from build123d import *

# Parameters (mm, degrees)
F0_R     = 15.6845
F0_R_2   = 11.499076
F1_DEPTH = 12.7
F2_R     = 17.145
F3_DEPTH = 5.08
F5_D     = 0.254


with BuildPart() as f1:
    # F0 (on Top) → F1 (new body)
    with BuildSketch(Plane.XY):
        Circle(F0_R)
        Circle(F0_R_2, mode=Mode.SUBTRACT)
    extrude(amount=F1_DEPTH)

    # F2 (on Top) → F3 (join)
    with BuildSketch(Plane.XY):
        Circle(F2_R)
    extrude(amount=F3_DEPTH)

    # F5 (through all)
    with Locations(Plane.XY.offset(5.08)):
        with Locations((0, 0)):
            Hole(F5_D / 2)


solid = f1.part
Build history of the part. All positions in model axes, mm. A direction names the side the tool comes from. Coordinates: 2 decimals unless noted, no trailing zeros. Order: outer loops, then holes, each group sorted by start corner. A loop starts at its lowest first (then second) coordinate and runs counter-clockwise, first axis right, second up. Notation, with made-up numbers: (60.5, -31.75) - (99.5, -31.75) arc R17 cw to (99.5, -25.75) - close; hole circle Ø1 at (-7, 3). An arc over 180 degrees is marked (long way). Put each result on its own line as item: value.
1. Saw through at A-A (z = 3.5). Write the cut outline in (x, y) (3 decimals).
Answer sheet:
outline: circle Ø34.29 at (0, 0); hole circle Ø0.254 at (0, 0)
2. Drop flat-ended pins along their axis: P1, Ø5, axis at x = -10, z = 6.5, coming from the -Y side; P2, Ø10.5, axis at x = 1, y = -3.5, coming from the +Z side; P3, Ø3, axis at y = -11, z = 2, coming from the +X side. Give the stop position or say it passes through.
Answer sheet:
P1: stops at y = -15.19
P2: stops at z = 5.08
P3: stops at x = 14.27
3. Saw through at B-B (y = 7). Write the cut outline in (x, z), and give its area (3 significant figures).
Answer sheet:
outline: (-15.65, 0) - (15.65, 0) - (15.65, 5.08) - (14.04, 5.08) - (14.04, 12.7) - (9.12, 12.7) - (9.12, 5.08) - (-9.12, 5.08) - (-9.12, 12.7) - (-14.04, 12.7) - (-14.04, 5.08) - (-15.65, 5.08) - close
area: 234 mm^2
4. Pull direction Y, two halves, no side cores. Call faces 3 (the face through (-2.493, -11.226, 8.837)), 4 (the face through (-1, 12, 12.7)), 5 (the face through (-3.4, -15.31, 8.84)): pulls with the +Y half, pulls with the -Y half, needs draft (parallel to the pull), parting line crosses it, or undercut.
Answer sheet:
face 3: undercut
face 4: needs draft
face 5: parting line crosses it
5. Probe line 1 along Y through (x, z) = (0, 8.25); line 2 along Z through (x, y) = (-4.5, -6.5). List the from-to ranges inside material, lowest first. Write a range as [from, to].
Answer sheet:
line 1: y = [-15.68, -11.5], [11.5, 15.68]
line 2: z = [0, 5.08]
6. Tool access for faces 1 (the face through (-0.2, 0.2, 0)), 2 (the face through (-0.2, 0.2, 5.08)): list every direction of +Z, -Z, +X, -X, +Y, -Y with a clear straight run to the whole face (end or side of a thin tool).
Answer sheet:
face 1: -Z, +X, -X, +Y, -Y
face 2: +Z
7. Saw through at D-D (y = -4). Write the cut outline in (x, z).
Answer sheet:
outline: (-16.67, 0) - (16.67, 0) - (16.67, 5.08) - (15.17, 5.08) - (15.17, 12.7) - (10.78, 12.7) - (10.78, 5.08) - (-10.78, 5.08) - (-10.78, 12.7) - (-15.17, 12.7) - (-15.17, 5.08) - (-16.67, 5.08) - close
8. Saw through at C-C (x = 13.5). Write the cut outline in (y, z).
Answer sheet:
outline: (-10.57, 0) - (10.57, 0) - (10.57, 5.08) - (7.98, 5.08) - (7.98, 12.7) - (-7.98, 12.7) - (-7.98, 5.08) - (-10.57, 5.08) - close
